from build123d import *

# Parameters (mm, degrees)
SKETCH2_R               = 1.2
CUT_EXTRUDE1_DEPTH      = 3.875
CUT_EXTRUDE1_DEPTH_BACK = 3.875
SKETCH3_W               = 5.75
SKETCH3_H               = 1.5
CUT_EXTRUDE2_DEPTH      = 6.5
SKETCH4_R               = 5
BOSS_EXTRUDE1_DEPTH     = 0.75


with BuildPart() as part:
    # Sketch1 → Revolve1 (revolve)
    with BuildSketch(Plane.XY):
        Polygon((0, 0), (1.5, 0), (1.5, 21.1), (2.875, 24.6), (2.875, 56.6), (0, 56.6), align=None)
    revolve(axis=Axis((0, 56.6, 0), (0, -1, 0)))

    # Sketch2 → Cut-Extrude1 (cut, two sides)
    with BuildSketch(Plane.XY) as cut_extrude1_sk:
        with Locations((0, 53.4)):
            Circle(SKETCH2_R)
    extrude(amount=CUT_EXTRUDE1_DEPTH, mode=Mode.SUBTRACT)
    extrude(cut_extrude1_sk.sketch, amount=-CUT_EXTRUDE1_DEPTH_BACK, mode=Mode.SUBTRACT)

    # Sketch3 → Cut-Extrude2 (cut)
    with BuildSketch(Plane(origin=(0, 56.6, 0), x_dir=(1, 0, 0), z_dir=(0, 1, 0))):
        Rectangle(SKETCH3_W, SKETCH3_H)
    extrude(amount=-CUT_EXTRUDE2_DEPTH, mode=Mode.SUBTRACT)

    # Sketch4 → Boss-Extrude1 (add)
    with BuildSketch(Plane(origin=(0, 47.6, 0), x_dir=(1, 0, 0), z_dir=(0, 1, 0))):
        Circle(SKETCH4_R)
    extrude(amount=BOSS_EXTRUDE1_DEPTH)


solid = part.part
Part model, mm, in its own coordinate system. A direction names the side the tool comes from. Coordinates: 2 decimals unless noted, no trailing zeros. Order: outer loops, then holes, each group sorted by start corner. A loop starts at its lowest first (then second) coordinate and runs counter-clockwise, first axis right, second up.
(1) Slice it at D-D, the plane y = 19. Write the cut outline in (x, z).
Check sheet entries:
outline: circle Ø3 at (0, 0)
(2) Slice it at A-A, the plane x = 0. Write the cut outline in (y, z) (3 decimals), and give its area (3 significant figures).
Check sheet entries:
outline: (0, -1.5) - (21.1, -1.5) - (24.6, -2.875) - (47.6, -2.875) - (47.6, -5) - (48.35, -5) - (48.35, -2.875) - (52.2, -2.875) - (52.2, -0.75) - (50.1, -0.75) - (50.1, 0.75) - (52.2, 0.75) - (52.2, 2.875) - (48.35, 2.875) - (48.35, 5) - (47.6, 5) - (47.6, 2.875) - (24.6, 2.875) - (21.1, 1.5) - (0, 1.5) - close; (54.6, -2.875) - (56.6, -2.875) - (56.6, -0.75) - (54.6, -0.75) - close; (54.6, 0.75) - (56.6, 0.75) - (56.6, 2.875) - (54.6, 2.875) - close
area: 246 mm2
(3) Tool access for faces 4 (the face through (-0.37, 36.26, 2.85)), 5 (the face through (1.11, 52.94, -1.8)), 6 (the face through (2.2, 48.35, 2.2)), 7 (the face through (-1.3, 52.7, -0.75)): list every direction of +Z, -Z, +X, -X, +Y, -Y with a clear straight run to the whole face (end or side of a thin tool).
Check sheet entries:
face 4: -Y
face 5: +Z, -Z
face 6: +Y
face 7: +X, -X, +Y
(4) Probe L1, parallel to Y at x = 4.25, z = 0.75; L2, parallel to Y at x = 0, z = 1.2; L3, parallel to X at y = 53.4, z = -1.95. List the from-to ranges inside material, lowest first.
Check sheet entries:
L1: y = 47.6 to 48.35
L2: y = 0 to 52.2, 54.6 to 56.6
L3: x = -2.11 to -1.2, 1.2 to 2.11
(5) Slice it at C-C, the plane y = 53.4. Write the cut outline in (x, z) (3 decimals), and give its area (3 significant figures).
Check sheet entries:
outline: (-2.775, -0.75) arc R2.875 ccw to (-1.2, -2.613) - (-1.2, -0.75) - close; (-2.775, 0.75) - (-1.2, 0.75) - (-1.2, 2.613) arc R2.875 ccw to start; (1.2, -2.613) arc R2.875 ccw to (2.775, -0.75) - (1.2, -0.75) - close; (1.2, 0.75) - (2.775, 0.75) arc R2.875 ccw to (1.2, 2.613) - close
area: 7.65 mm2
(6) Pin check, flat tips, straight feed: pin 1 Ø3 at (x, y) = (0, 53.4) entering from +Z (3 decimals); pin 2 Ø6 at (x, y) = (3.5, 40) entering from -Z; pin 3 Ø3 at (y, z) = (48.5, -2.5) entering from -X. Stop position of each tip, or through.
Check sheet entries:
pin 1: stops at z = 2.875
pin 2: stops at z = -2.83
pin 3: stops at x = -4.9
(7) Pull direction X, two halves, no side cores. Call faces 1 (the face through (-1.08, 47.97, 4.88)), 2 (the face through (0, 50.1, 0)), 3 (the face through (1.11, 52.94, 1.8)): pulls with the +X half, pulls with the -X half, needs draft (parallel to the pull), parting line crosses it, or undercut.
Check sheet entries:
face 1: parting line crosses it
face 2: needs draft
face 3: undercut
(8) Slice it at B-B, the plane z = 0. Write the cut outline in (x, y) (3 decimals).
Check sheet entries:
outline: (-5, 47.6) - (-2.875, 47.6) - (-2.875, 24.6) - (-1.5, 21.1) - (-1.5, 0) - (1.5, 0) - (1.5, 21.1) - (2.875, 24.6) - (2.875, 47.6) - (5, 47.6) - (5, 48.35) - (2.875, 48.35) - (2.875, 50.1) - (-2.875, 50.1) - (-2.875, 48.35) - (-5, 48.35) - close
